Geometry check sheet. Reference: drawing and pictorial views, mm from the part's lowest x, y, z. Round coordinates to 2 decimals unless told otherwise and drop trailing zeros. Order: outer loops, then holes, each group sorted by start corner. A loop starts at its lowest first (then second) coordinate and runs counter-clockwise, first axis right, second up.
(1) Go/stop test with a flat-tipped pin: pin 1 (2.5 mm diameter, centred on x = 35.25, z = 35.25, fed in from +Y). Record where the tip stops, or that it passes through.
(2) Sectioned sample at B-B (x = 35.25). Record the boundary of the cut face in (y, z).
(3) Material ranges on line 1 along Z through (x, y) = (4.75, 0.6); line 2 along X through (y, z) = (0.7, 4.5); line 3 along Z through (x, y) = (38.5, 0.7), recorded low to high.
(4) Sectioned sample at C-C (y = 0.4). Record the boundary of the cut face in (x, z).
(5) Sectioned sample at A-A (z = 35.25). Record the boundary of the cut face in (x, y), plus the area to 3 significant figures.
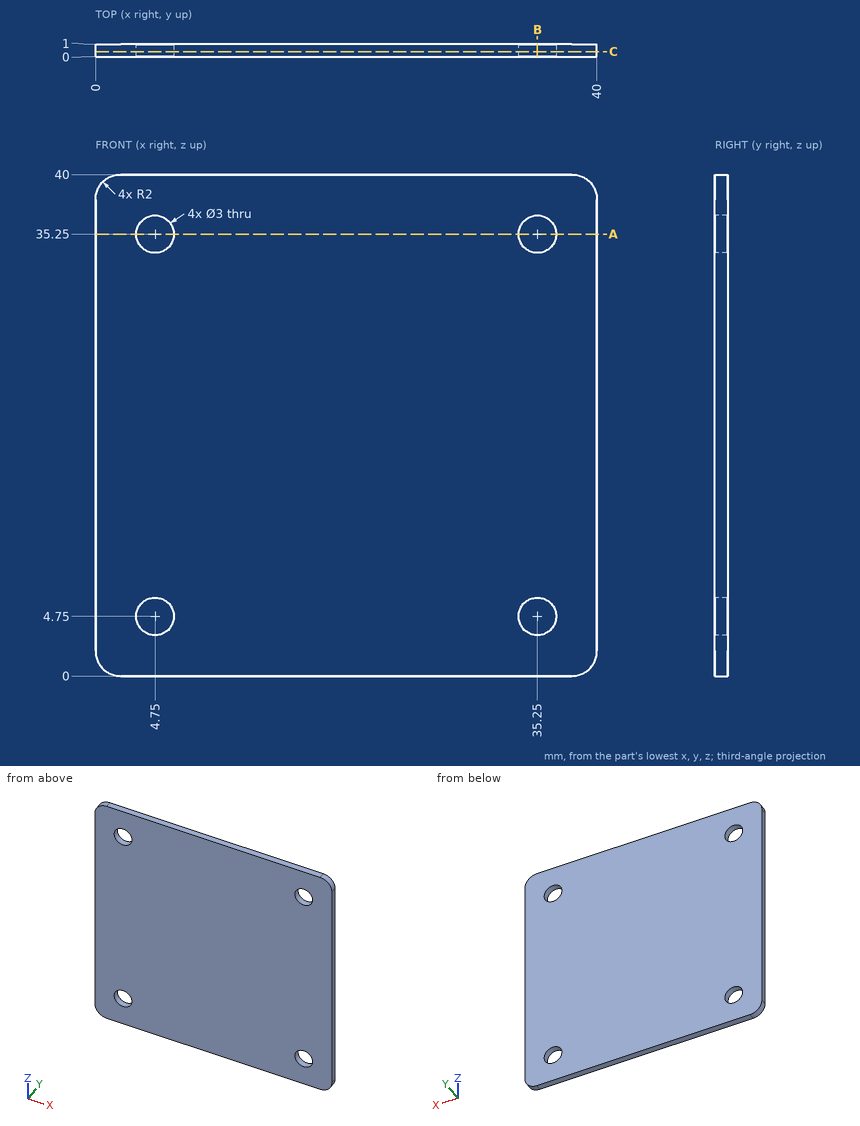
Answer below:
1. pin 1: passes through
2. outline: (0, 0) - (1, 0) - (1, 3.25) - (0, 3.25) - close; (0, 6.25) - (1, 6.25) - (1, 33.75) - (0, 33.75) - close; (0, 36.75) - (1, 36.75) - (1, 40) - (0, 40) - close
3. line 1: z = 0 to 3.25, 6.25 to 33.75, 36.75 to 40
3. line 2: x = 0 to 3.27, 6.23 to 33.77, 36.73 to 40
3. line 3: z = 0.06 to 39.94
4. outline: (0, 2) arc R2 ccw to (2, 0) - (38, 0) arc R2 ccw to (40, 2) - (40, 38) arc R2 ccw to (38, 40) - (2, 40) arc R2 ccw to (0, 38) - close; hole circle Ø3 at (4.75, 4.75); hole circle Ø3 at (4.75, 35.25); hole circle Ø3 at (35.25, 4.75); hole circle Ø3 at (35.25, 35.25)
5. outline: (0, 0) - (3.25, 0) - (3.25, 1) - (0, 1) - close; (6.25, 0) - (33.75, 0) - (33.75, 1) - (6.25, 1) - close; (36.75, 0) - (40, 0) - (40, 1) - (36.75, 1) - close
5. area: 34.0 mm2
